Source: CAD feature listing. Evaluate the final solid. Frame: model axes, mm. A direction names the side the tool comes from. Give positions to 0.01 mm unless a question says otherwise; leave off trailing zeros. Loops run counter-clockwise (first coordinate to the right, second up) from the corner with the lowest first, then second, coordinate; pieces in that order, holes last. Notation, with made-up numbers: M 79.25,-11.75 L 94.25,-11.75 A38 ccw 94.25,27.25 Z; hole C -2.75,67.25 d1. An arc over 180 degrees is marked long. Put each result on its own line as item: value. Start each with the question number.
```python
from build123d import *

# Parameters (mm, degrees)
SKETCH1_W           = 35
SKETCH1_H           = 56
SKETCH1_R           = 1
SKETCH1_R_2         = 0.5
BOSS_EXTRUDE1_DEPTH = 1.2
FILLET1_R           = 1
SKETCH2_W           = 34
SKETCH2_H           = 45.5
BOSS_EXTRUDE2_DEPTH = 2.4
CUT_EXTRUDE1_DEPTH  = 0.1


with BuildPart() as part:
    # Sketch1 → Boss-Extrude1 (new body)
    with BuildSketch(Plane(origin=(0, 0, 0), x_dir=(1, 0, 0), z_dir=(0, 1, 0))):
        Rectangle(SKETCH1_W, SKETCH1_H)
        with Locations((-14.7, 25.5)):
            Circle(SKETCH1_R, mode=Mode.SUBTRACT)
        with Locations((14.7, 25.5)):
            Circle(SKETCH1_R, mode=Mode.SUBTRACT)
        with Locations((-14.7, -25.5)):
            Circle(SKETCH1_R, mode=Mode.SUBTRACT)
        with Locations((14.7, -25.5)):
            Circle(SKETCH1_R, mode=Mode.SUBTRACT)
        with Locations((-9, 26.8)):
            Circle(SKETCH1_R_2, mode=Mode.SUBTRACT)
        with Locations((-6.46, 26.8)):
            Circle(SKETCH1_R_2, mode=Mode.SUBTRACT)
        with Locations((-3.92, 26.8)):
            Circle(SKETCH1_R_2, mode=Mode.SUBTRACT)
        with Locations((-1.38, 26.8)):
            Circle(SKETCH1_R_2, mode=Mode.SUBTRACT)
        with Locations((1.16, 26.8)):
            Circle(SKETCH1_R_2, mode=Mode.SUBTRACT)
        with Locations((3.7, 26.8)):
            Circle(SKETCH1_R_2, mode=Mode.SUBTRACT)
        with Locations((6.24, 26.8)):
            Circle(SKETCH1_R_2, mode=Mode.SUBTRACT)
        with Locations((8.78, 26.8)):
            Circle(SKETCH1_R_2, mode=Mode.SUBTRACT)
    extrude(amount=BOSS_EXTRUDE1_DEPTH)

    # Fillet1
    fillet1_edges = [part.edges().sort_by_distance(p)[0] for p in [
        (17.5, 0.6, 28),
        (-17.5, 0.6, 28),
        (-17.5, 0.6, -28),
        (17.5, 0.6, -28),
    ]]
    fillet(fillet1_edges, radius=FILLET1_R)

    # Sketch2 → Boss-Extrude2 (add)
    with BuildSketch(Plane(origin=(0, 1.2, 0), x_dir=(1, 0, 0), z_dir=(0, 1, 0))):
        with Locations((0, 0.02)):
            Rectangle(SKETCH2_W, SKETCH2_H)
    extrude(amount=BOSS_EXTRUDE2_DEPTH)

    # Sketch3 → Cut-Extrude1 (cut)
    with BuildSketch(Plane(origin=(0, 3.6, 0), x_dir=(1, 0, 0), z_dir=(0, 1, 0))):
        Polygon((-16.27, 22.04), (16.27, 22.04), (16.27, -20.43), (14.4, -20.43), (14.4, -22.73), (-14.4, -22.73), (-14.4, -20.43), (-16.27, -20.43), align=None)
    extrude(amount=-CUT_EXTRUDE1_DEPTH, mode=Mode.SUBTRACT)


solid = part.part
```
1. Set-up query: faces 4 (the face through (17, 2, 0)), 5 (the face through (0, 2, -22.77)), 6 (the face through (-14.24, 0.59, 26.39)). Return all of +Z, -Z, +X, -X, +Y, -Y with unobstructed straight access to the full face (end or side cutting, diameter ignored); none if empty.
2. Section A-A, the plane x = -12.5. Output: boundary loops of the cut face in (y, z).
3. Section B-B, the plane z = 5. Output: boundary loops of the cut face in (x, y).
4. Contact query for flat-ended pins moving along their axis: pin 1 (8 mm diameter, centred on x = 12, z = -2, fed in from +Y); pin 2 (4 mm diameter, centred on x = -9, z = -1.5, fed in from -Y); pin 3 (1.9 mm diameter, centred on x = 0, y = 3, fed in from +Z); pin 4 (3 mm diameter, centred on x = 14.7, z = -25.5, fed in from +Y). Output: stop coordinate, or through.
5. Ray query, line 1 (X direction, y = 0.8, z = -25.5); line 2 (Z direction, x = 14.7, y = 0.85); line 3 (Z direction, x = 6.24, y = 0.65). Return the intervals inside material, ascending.
6. Section C-C, the plane y = 2.05. Output: boundary loops of the cut face in (x, z), plus the area to 3 significant figures.
7. Pull-direction query (X, two-part tool) for faces 1 (the face through (0, 3.5, 0)), 2 (the face through (0, 0, 0)), 3 (the face through (17.199, 0.608, 27.715)); classes: released by +X, released by -X, zero draft, split by the parting line, or undercut.
Results found:
1. face 4: +Z, -Z, +X, +Y
1. face 5: -Z, +X, -X, +Y
1. face 6: +Y, -Y
2. outline: M 0,-28 L 1.2,-28 L 1.2,-22.77 L 3.6,-22.77 L 3.6,-22.04 L 3.5,-22.04 L 3.5,22.73 L 1.2,22.73 L 1.2,28 L 0,28 Z
3. outline: M -17.5,0 L 17.5,0 L 17.5,1.2 L 17,1.2 L 17,3.6 L 16.27,3.6 L 16.27,3.5 L -16.27,3.5 L -16.27,3.6 L -17,3.6 L -17,1.2 L -17.5,1.2 Z
4. pin 1: y = 3.5
4. pin 2: y = 0
4. pin 3: z = 22.73
4. pin 4: y = 1.2
5. line 1: -17.5 to -15.7, -13.7 to 13.7, 15.7 to 17.5
5. line 2: -28 to -26.5, -24.5 to 24.5, 26.5 to 28
5. line 3: -28 to -27.3, -26.3 to 28
6. outline: M -17,-22.77 L 17,-22.77 L 17,22.73 L -17,22.73 Z
6. area: 1,550 mm²
7. face 1: undercut
7. face 2: zero draft
7. face 3: released by +X
